Autodesk Inventor part; units mm, degrees
ref_plane "YZ Plane" through (0, 0, 0) normal (1, 0, 0) x (0, 1, 0)
ref_plane "XZ Plane" through (0, 0, 0) normal (0, 1, 0) x (-1, 0, 0)
ref_plane "XY Plane" through (0, 0, 0) normal (0, 0, 1) x (1, 0, 0)
sketch "Sketch1" plane through (0, 0, 0) normal (0, 1, 0) x (-1, 0, 0)
  line L0 (12.5, 25) -> (-12.5, 25)
  line L1 (-11, -25) -> (11, -25)
  line L2 (15, -21) -> (15, 22.5)
  line L3 (22.1598, 0) -> (-22.1598, 0) construction
  line L4 (0, -36.0977) -> (0, 35.787) construction
  arc A0 (-15, -21) -> (-11, -25) centre (-11, -21) ccw
  arc A1 (11, -25) -> (15, -21) centre (11, -21) ccw
  arc A2 (-12.5, 25) -> (-15, 22.5) centre (-12.5, 22.5) ccw
  arc A3 (15, 22.5) -> (12.5, 25) centre (12.5, 22.5) ccw
  line L5 (-15, 22.5) -> (-15, -21)
  point P0 (0, 0)
  point P1 (15, 25)
  point P2 (-15, -25)
  point P3 (-15, 25)
  point P4 (15, -25)
  point P5 (-15, 0)
  dimension "d6" = 15
  dimension "d10" = 4
  dimension "d11" = 2.5
  dimension "d15" = 15
  dimension "d35" = 50
extrude "Extrusion1" add sketch "Sketch1" along normal blind 1.6
sketch "Sketch2" plane through (0, 1.6, 0) normal (0, 1, 0) x (1, 0, 0)
  line L0 (15, -22.5) -> (15, 21)
  line L1 (-15, 21) -> (-15, -22.5)
  line L2 (-12.5, -25) -> (12.5, -25)
  arc A0 (15, 21) -> (11, 25) centre (11, 21) ccw
  arc A1 (-11, 25) -> (-15, 21) centre (-11, 21) ccw
  point P0 (0, 0)
  point P1 (-11, -8.5)
  point P2 (11, -7)
  dimension "d36" = 28
  dimension "d37" = 1.5
hole "Hole1" at (11, 1.6, -21) at (-11, 1.6, -21) at (-11, 1.6, 8.5) at (11, 1.6, 7) direction (0, -1, 0) diameter 3.4 end through all
sketch "Sketch3" plane through (0, 1.6, 0) normal (0, 1, 0) x (1, 0, 0)
  line L0 (4.3, -1.51) -> (-4.3, -1.51)
  line L1 (-4.3, -1.51) -> (-4.3, 15.75)
  line L2 (-4.3, 15.75) -> (4.3, 15.75)
  line L3 (4.3, 15.75) -> (4.3, -1.51)
  line L4 (0, 35) -> (0, -35) construction
  line L5 (11, 25) -> (-11, 25)
  point P0 (0, 0)
  dimension "d29" = 9.25
  dimension "d30" = 8.6
  dimension "d31" = 17.26
extrude "Extrusion2" cut sketch "Sketch3" against normal through all
sketch "Sketch5" plane through (0, 1.6, 0) normal (0, 1, 0) x (1, 0, 0)
  line L0 (15, -22.5) -> (15, 21)
  arc A0 (12, 8.5) -> (12, 3.5) centre (12, 6) ccw
  line L1 (11, 25) -> (-11, 25)
  arc A1 (15, 0.5) -> (12, 3.5) centre (12, 0.5) ccw
  arc A2 (12, 8.5) -> (15, 11.5) centre (12, 11.5) ccw
  point P0 (0, 0)
  dimension "d47" = 5
  dimension "d48" = 3
  dimension "d49" = 19
extrude "Extrusion3" cut sketch "Sketch5" against normal through all
properties part number "sensor_pcb"
Could you check a few things on this model? Use its own coordinates, in mm. A direction names the side the tool comes from. Give positions to 0.01 mm unless a question says otherwise; leave off trailing zeros. Order: outer loops, then holes, each group sorted by start corner. A loop starts at its lowest first (then second) coordinate and runs counter-clockwise, first axis right, second up.
1. Which directions (+Z, -Z, +X, -X, +Y, -Y) give clear straight access to the entire face, cutting with the end or side of a thin tool? Please do faces 5 (the cylindrical face through (14.1, 0.81, -9.36)), 6 (the flat face through (15, 1, -16)), 7 (the flat face through (0, 1, 1.51)).
Answers below:
face 5: +X, +Y, -Y
face 6: +Z, -Z, +X, +Y, -Y
face 7: +Y, -Y
2. Suppose I cut it at A-A (z = -6). Write out the boundary of the cut face in (x, y).
Answers below:
outline: (-15, 0) - (-4.3, 0) - (-4.3, 1.6) - (-15, 1.6) - close; (4.3, 0) - (9.5, 0) - (9.5, 1.6) - (4.3, 1.6) - close
3. Suppose I cut it at D-D (x = -10). Write out the boundary of the cut face in (y, z).
Answers below:
outline: (0, -25) - (1.6, -25) - (1.6, -22.37) - (0, -22.37) - close; (0, -19.63) - (1.6, -19.63) - (1.6, 7.13) - (0, 7.13) - close; (0, 9.87) - (1.6, 9.87) - (1.6, 25) - (0, 25) - close
4. Suppose I cut it at B-B (y = 0.65). Write out the boundary of the cut face in (x, z), plus the area to 3 significant figures.
Answers below:
outline: (-15, -21) arc R4 ccw to (-11, -25) - (11, -25) arc R4 ccw to (15, -21) - (15, -11.5) arc R3 ccw to (12, -8.5) arc R2.5 cw to (12, -3.5) arc R3 ccw to (15, -0.5) - (15, 22.5) arc R2.5 ccw to (12.5, 25) - (-12.5, 25) arc R2.5 ccw to (-15, 22.5) - close; hole circle Ø3.4 at (-11, -21); hole circle Ø3.4 at (-11, 8.5); hole (-4.3, -15.75) - (4.3, -15.75) - (4.3, 1.51) - (-4.3, 1.51) - close; hole circle Ø3.4 at (11, -21); hole circle Ø3.4 at (11, 7)
area: 1,280 mm2
5. Suppose I cut it at C-C (x = -1.25). Write out the boundary of the cut face in (y, z).
Answers below:
outline: (0, -25) - (1.6, -25) - (1.6, -15.75) - (0, -15.75) - close; (0, 1.51) - (1.6, 1.51) - (1.6, 25) - (0, 25) - close
6. Thinking about a two-plate mould opening in Z: for faces 1 (the cylindrical face through (-13.859, 0.789, -23.797)), 2 (the flat face through (-4.3, 1, -7)), 3 (the cylindrical face through (-14.248, 0.789, 24.287)), 4 (the flat face through (0, 0, 6)), which applies, +Z half, -Z half, draft (parallel to the pull), parting line (faces both ways), or undercut?
Answers below:
face 1: -Z half
face 2: undercut
face 3: +Z half
face 4: draft
7. I need wall thicknesses on L1, parallel to X at y = 0.85, z = -21; L2, parallel to X at y = 0.6, z = -21.5; L3, parallel to Z at x = 11, y = 0.8. Which ranges of each line are inside material? Lowest first, please.
Answers below:
L1: x = -15 to -12.7, -9.3 to 9.3, 12.7 to 15
L2: x = -14.97 to -12.62, -9.38 to 9.38, 12.62 to 14.97
L3: z = -25 to -22.7, -19.3 to -8.29, -3.71 to 5.3, 8.7 to 25
